Build history of the part. All positions in model axes, mm. A direction names the side the tool comes from. Round coordinates to 2 decimals unless told otherwise and drop trailing zeros. Write each loop counter-clockwise with the first axis right and the second up, starting at its lowest first coordinate (ties: lowest second). Pieces come first, ordered by that corner, then holes.
from build123d import *

# Parameters (mm, degrees)
SKETCH1_W               = 190.5
SKETCH1_H               = 25.4
SKETCH1_R               = 6.35
BOSS_EXTRUDE1_DEPTH     = 3.175
SKETCH2_W               = 146.05
SKETCH2_H               = 3.175
BOSS_EXTRUDE2_DEPTH     = 47.625
BOSS_EXTRUDE2_2_DEPTH   = 47.625
SKETCH3_W               = 146.05
SKETCH3_H               = 25.4
BOSS_EXTRUDE4_DEPTH     = 6.35
SKETCH4_W               = 3.175
SKETCH4_H               = 25.4
BOSS_EXTRUDE5_DEPTH     = 41.275
SKETCH5_W               = 6.35
SKETCH5_H               = 25.4
CUT_EXTRUDE1_DEPTH      = 165.45
SKETCH7_W               = 146.05
SKETCH7_H               = 31.75
BOSS_EXTRUDE7_DEPTH     = 3.175
FILLET1_R               = 10
SKETCH8_R               = 3.05
CUT_EXTRUDE2_DEPTH      = 3.175
SKETCH9_W               = 6.35
SKETCH9_H               = 38.1
SKETCH9_H_2             = 50.8
BOSS_EXTRUDE8_DEPTH     = 12.7
SKETCH10_R              = 3.175
CUT_EXTRUDE3_DEPTH      = 12.7
SKETCH11_W              = 6.35
SKETCH11_H              = 25.4
BOSS_EXTRUDE9_DEPTH     = 12.7
SKETCH12_R              = 3.175
CUT_EXTRUDE4_DEPTH      = 12.7
SKETCH13_W              = 28.740264125
SKETCH13_H              = 146.120317421
CUT_EXTRUDE5_DEPTH      = 50.8
CUT_EXTRUDE5_DEPTH_BACK = 50.8


with BuildPart() as part:
    # Sketch1 → Boss-Extrude1 (new body)
    with BuildSketch(Plane(origin=(0, 0, 0), x_dir=(0, 0, -1), z_dir=(1, 0, 0))):
        with Locations((-50.270833333, 2.116666667)):
            Rectangle(SKETCH1_W, SKETCH1_H)
        with Locations((32.279166667, 2.116666667)):
            Circle(SKETCH1_R, mode=Mode.SUBTRACT)
        with Locations((-132.820833333, 2.116666667)):
            Circle(SKETCH1_R, mode=Mode.SUBTRACT)
    extrude(amount=BOSS_EXTRUDE1_DEPTH)



with BuildPart() as body_2:
    # Sketch2 → Boss-Extrude2 (new body)
    with BuildSketch(Plane(origin=(3.175, 0, 0), x_dir=(0, 0, -1), z_dir=(1, 0, 0))):
        with Locations((-50.270833333, 16.404166667)):
            Rectangle(SKETCH2_W, SKETCH2_H)
    extrude(amount=BOSS_EXTRUDE2_DEPTH)


with BuildPart() as body_3:
    # Sketch2 → Boss-Extrude2 2 (new body)
    with BuildSketch(Plane(origin=(3.175, 0, 0), x_dir=(0, 0, -1), z_dir=(1, 0, 0))):
        with Locations((-50.270833333, -12.170833333)):
            Rectangle(SKETCH2_W, SKETCH2_H)
    extrude(amount=BOSS_EXTRUDE2_2_DEPTH)


with BuildPart() as part_1:
    add(part.part)

    add(body_2.part)  # Boss-Extrude4 merges body 2

    add(body_3.part)  # Boss-Extrude4 merges body 3
    # Sketch3 → Boss-Extrude4 (add)
    with BuildSketch(Plane(origin=(3.175, 0, 0), x_dir=(0, 0, -1), z_dir=(1, 0, 0))):
        with Locations((-50.270833333, 2.116666667)):
            Rectangle(SKETCH3_W, SKETCH3_H)
    extrude(amount=BOSS_EXTRUDE4_DEPTH)

    # Sketch4 → Boss-Extrude5 (add)
    with BuildSketch(Plane(origin=(9.525, 0, 0), x_dir=(0, 0, -1), z_dir=(1, 0, 0))):
        with Locations((-121.708333333, 2.116666667)):
            Rectangle(SKETCH4_W, SKETCH4_H)
        with Locations((21.166666667, 2.116666667)):
            Rectangle(SKETCH4_W, SKETCH4_H)
    extrude(amount=BOSS_EXTRUDE5_DEPTH)

    # Sketch5 → Cut-Extrude1 (cut)
    with BuildSketch(Plane.XY.offset(123.295833333)):
        with Locations((12.7, 2.116666667)):
            Rectangle(SKETCH5_W, SKETCH5_H)
    extrude(amount=-CUT_EXTRUDE1_DEPTH, mode=Mode.SUBTRACT)

    # Sketch7 → Boss-Extrude7 (add)
    with BuildSketch(Plane(origin=(50.8, 0, 0), x_dir=(0, 0, -1), z_dir=(1, 0, 0))):
        with Locations((-50.270833333, 2.116666667)):
            Rectangle(SKETCH7_W, SKETCH7_H)
    extrude(amount=BOSS_EXTRUDE7_DEPTH)

    # Fillet1
    fillet1_edges = [part_1.edges().sort_by_distance(p)[0] for p in [
        (53.975, 2.116666667, 123.295833333),
        (53.975, -13.758333333, 50.270833333),
        (53.975, 2.116666667, -22.754166667),
        (53.975, 17.991666667, 50.270833333),
    ]]
    fillet(fillet1_edges, radius=FILLET1_R)

    # Sketch8 → Cut-Extrude2 (cut)
    with BuildSketch(Plane.XZ.offset(13.758333333)):
        with Locations((28.575, 56.120833333)):
            Circle(SKETCH8_R)
    extrude(amount=-CUT_EXTRUDE2_DEPTH, mode=Mode.SUBTRACT)

    # Sketch9 → Boss-Extrude8 (add)
    with BuildSketch(Plane.XZ.offset(13.758333333)):
        with Locations((26.541679323, 97.895833333)):
            Rectangle(SKETCH9_W, SKETCH9_H)
        with Locations((26.541679323, 8.995833333)):
            Rectangle(SKETCH9_W, SKETCH9_H_2)
    extrude(amount=BOSS_EXTRUDE8_DEPTH)

    # Sketch10 → Cut-Extrude3 (cut)
    with BuildSketch(Plane(origin=(29.716679323, 0, 0), x_dir=(0, 0, -1), z_dir=(1, 0, 0))):
        with Locations((-97.895833333, -20.108333333)):
            Circle(SKETCH10_R)
        with Locations((-8.995833333, -20.108333333)):
            Circle(SKETCH10_R)
    extrude(amount=-CUT_EXTRUDE3_DEPTH, mode=Mode.SUBTRACT)

    # Sketch11 → Boss-Extrude9 (add)
    with BuildSketch(Plane(origin=(0, 17.991666667, 0), x_dir=(1, 0, 0), z_dir=(0, 1, 0))):
        with Locations((26.54, -49.945833333)):
            Rectangle(SKETCH11_W, SKETCH11_H)
    extrude(amount=BOSS_EXTRUDE9_DEPTH)

    # Sketch12 → Cut-Extrude4 (cut)
    with BuildSketch(Plane(origin=(29.715, 0, 0), x_dir=(0, 0, -1), z_dir=(1, 0, 0))):
        with Locations((-49.945833333, 24.341666667)):
            Circle(SKETCH12_R)
    extrude(amount=-CUT_EXTRUDE4_DEPTH, mode=Mode.SUBTRACT)

    # Sketch13 → Cut-Extrude5 (cut, two sides)
    with BuildSketch(Plane.XZ.offset(13.758333333)) as cut_extrude5_sk:
        with Locations((41.13133077, 50.235674622)):
            Rectangle(SKETCH13_W, SKETCH13_H)
    extrude(amount=CUT_EXTRUDE5_DEPTH, mode=Mode.SUBTRACT)
    extrude(cut_extrude5_sk.sketch, amount=-CUT_EXTRUDE5_DEPTH_BACK, mode=Mode.SUBTRACT)


solid = part_1.part
1) Slice it at D-D (x = 6.5). Write the cut outline in (y, z), plus the area to 3 significant figures.
Results:
outline: (-13.76, -22.75) - (17.99, -22.75) - (17.99, 123.3) - (-13.76, 123.3) - close
area: 4,640 mm2
2) Pin check, flat tips, straight feed: pin 1 Ø2 at (x, y) = (23.5, 23.5) entering from -Z; pin 2 Ø3.5 at (x, y) = (25, -21) entering from +Z; pin 3 Ø8 at (x, z) = (18, 75.5) entering from +Y; pin 4 Ø5 at (y, z) = (-12.5, 66) entering from -X. Stop position of each tip, or through.
Results:
pin 1: stops at z = 37.25
pin 2: stops at z = 116.95
pin 3: stops at y = 17.99
pin 4: stops at x = 0
3) Slice it at A-A (x = 19.75). Write the cut outline in (y, z), plus the area to 3 significant figures.
Results:
outline: (-13.76, -22.75) - (17.99, -22.75) - (17.99, 123.3) - (-13.76, 123.3) - close; hole (-10.58, -19.58) - (14.82, -19.58) - (14.82, 120.12) - (-10.58, 120.12) - close
area: 1,090 mm2
4) Wall check: L1, parallel to Y at x = 14.5, z = 89; L2, parallel to Z at x = 19.75, y = 8; L3, parallel to Y at x = 23.75, z = 3. Give the ranges that are in metal, low to high.
Results:
L1: y = -13.76 to -10.58, 14.82 to 17.99
L2: z = -22.75 to -19.58, 120.12 to 123.3
L3: y = -26.46 to -10.58, 14.82 to 17.99
5) Slice it at B-B (z = 43.5). Write the cut outline in (x, y) (3 decimals).
Results:
outline: (0, -10.583) - (3.175, -10.583) - (3.175, -13.758) - (26.761, -13.758) - (26.761, -10.583) - (9.525, -10.583) - (9.525, 14.817) - (26.761, 14.817) - (26.761, 30.692) - (23.365, 30.692) - (23.365, 17.992) - (3.175, 17.992) - (3.175, 14.817) - (0, 14.817) - close
6) Slice it at C-C (z = 76.5). Write the cut outline in (x, y) (3 decimals), plus the area to 3 significant figures.
Results:
outline: (0, -10.583) - (3.175, -10.583) - (3.175, -13.758) - (26.761, -13.758) - (26.761, -10.583) - (9.525, -10.583) - (9.525, 14.817) - (26.761, 14.817) - (26.761, 17.992) - (3.175, 17.992) - (3.175, 14.817) - (0, 14.817) - close
area: 392 mm2
7) Which spindle directions (+Z, -Z, +X, -X, +Y, -Y) get a long thin tool onto all of the face, cutting with end or side? Do faces 1 (the flat face through (25, 24, 62.646)), 2 (the flat face through (25, -20, 34.396)), 3 (the flat face through (3.175, -12, 51)), 4 (the flat face through (17, 2, 123.296)). Say none if no direction does.
Results:
face 1: +Z, +X, -X, +Y
face 2: +X, -X, -Y
face 3: +Z, -Z, -X, -Y
face 4: +Z, +X, +Y, -Y
8) Mould opens along X. For faces 5 (the flat face through (21, 2, 120.121)), 6 (the flat face through (23.367, -24, 9)), 7 (the flat face through (15.875, 2, -21)) say: released by +X, released by -X, zero draft, split by the parting line, or undercut.
Results:
face 5: zero draft
face 6: released by -X
face 7: undercut
